Read the model definition and answer for the solid it produces. Units are mm, in the model's axes. A direction names the side the tool comes from. Coordinates: 2 decimals unless noted, no trailing zeros. Write each loop counter-clockwise with the first axis right and the second up, starting at its lowest first coordinate (ties: lowest second). Pieces come first, ordered by that corner, then holes.
1) The part is cut by section A-A (x = -145.5). Determine the outline of the cut face in (y, z) (3 decimals), then the cut area to 3 significant figures.
2) Find the intervals of material crossed by line 1 (Z direction, x = -10, y = -43); line 2 (Y direction, x = -126, z = 153.5) (3 decimals); line 3 (Y direction, x = -82, z = 149.5) (3 decimals), in increasing order.
3) The part is cut by section C-C (y = -5.5). Determine the outline of the cut face in (x, z).
4) The part is cut by section B-B (z = 141.5). Determine the outline of the cut face in (x, y) (3 decimals).
5) Which of the six approach directions +Z, -Z, +X, -X, +Y, -Y give full straight-line access (tool end or side, diameter ignored) to faces 1 (the face through (-78, -75, 153.924)), 2 (the face through (-153, -39, 153))?
6) Each of these flat-tipped pins is pushed along its axis until it touches: pin 1 Ø5 at (x, z) = (-82, 146.5) entering from -Y (3 decimals); pin 2 Ø10 at (x, y) = (-111, -22.5) entering from -Z; pin 3 Ø2.5 at (x, y) = (-68.5, -75) entering from -Z; pin 4 Ø8 at (x, z) = (-70, 151) entering from -Y. Where does it stop, or does it pass through?
7) The part is cut by section D-D (x = -11). Determine the outline of the cut face in (y, z) (3 decimals), then the cut area to 3 significant figures.
from build123d import *

# Parameters (mm, degrees)
F1_DEPTH = 76.2
F2_W     = 153.924
F2_H     = 153.924
F3_DEPTH = 3.175
F4_W     = 149.86
F4_H     = 149.86
F5_DEPTH = 63.5
F7_DEPTH = 76.201


# Not quite as in the source:
# - a feature names something its author has since deleted; it is built from what else it names


with BuildPart() as f1:
    # F0 (on Front) → F1 (new body)
    with BuildSketch(Plane.XZ):
        Polygon((0, 139.7), (0, 158.75), (-158.75, 158.75), (-158.75, 0), (-139.7, 0), (-139.7, 139.7), align=None)
    extrude(amount=F1_DEPTH)

    # F2 (on face) → F3 (cut)
    with BuildSketch(Plane.XZ.offset(76.2)):
        with Locations((-76.962, 76.962)):
            Rectangle(F2_W, F2_H)
    extrude(amount=-F3_DEPTH, mode=Mode.SUBTRACT)

    # F4 (on face) → F5 (cut)
    with BuildSketch(Plane.XZ.offset(73.025)):
        with Locations((-74.93, 74.93)):
            Rectangle(F4_W, F4_H)
    extrude(amount=-F5_DEPTH, mode=Mode.SUBTRACT)

    # F6 (on face) → F7 (cut, through all)
    with BuildSketch(Plane.XZ.offset(76.2)):
        Polygon((-139.7, 139.7), (-158.75, 158.75), (-158.75, 0), (-139.7, 0), align=None)
    extrude(amount=-F7_DEPTH, mode=Mode.SUBTRACT)


solid = f1.part
Reported:
1. outline: (-76.2, 153.924) - (-73.025, 153.924) - (-73.025, 149.86) - (-9.525, 149.86) - (-9.525, 145.5) - (0, 145.5) - (0, 158.75) - (-76.2, 158.75) - close
1. area: 706 mm2
2. line 1: z = 149.86 to 158.75
2. line 2: y = -73.025 to 0
2. line 3: y = -9.525 to 0
3. outline: (-158.75, 158.75) - (-139.7, 139.7) - (0, 139.7) - (0, 158.75) - close
4. outline: (-141.5, -9.525) - (0, -9.525) - (0, 0) - (-141.5, 0) - close
5. face 1: -Z, +X, -X, -Y
5. face 2: -Z, -X, +Y, -Y
6. pin 1: stops at y = -9.525
6. pin 2: stops at z = 149.86
6. pin 3: stops at z = 153.92
6. pin 4: stops at y = -76.2
7. outline: (-76.2, 153.924) - (-73.025, 153.924) - (-73.025, 149.86) - (-9.525, 149.86) - (-9.525, 139.7) - (0, 139.7) - (0, 158.75) - (-76.2, 158.75) - close
7. area: 761 mm2
